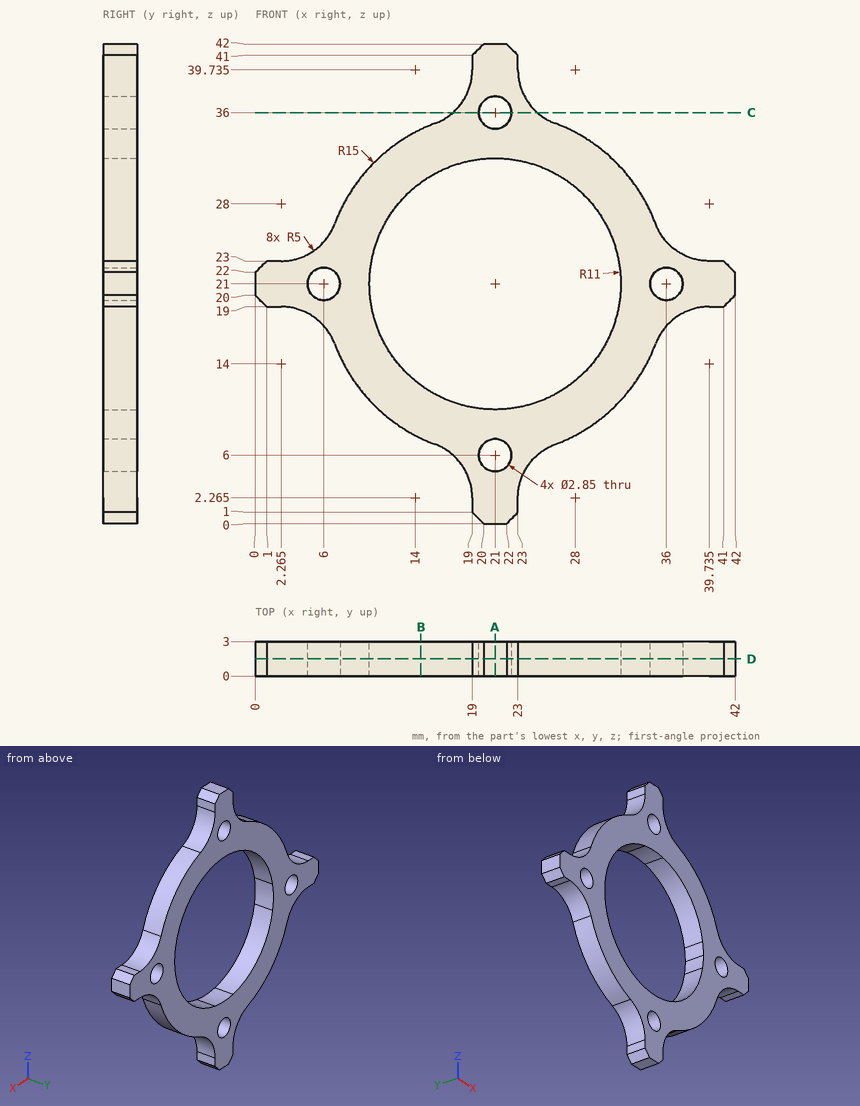
For this review, use the dimensioned drawing (mm, ordinates from the lowest corner) and the shaded views. Give positions to 0.01 mm unless a question says otherwise; leave off trailing zeros. Loops run counter-clockwise (first coordinate to the right, second up) from the corner with the lowest first, then second, coordinate; pieces in that order, holes last.
Item 1: Take a section at A-A, the plane x = 21. State the section outline as (y, z) points (3 decimals).
Item 2: For line 1 along X through (y, z) = (2.4, 21) (3 decimals); line 2 along X through (y, z) = (2.05, 22.5), list the stretches that pass through material, from the lowest coordinate up.
Item 3: Take a section at B-B, the plane x = 14.5. State the section outline as (y, z) points, and give its area (3 significant figures).
Item 4: Take a section at D-D, the plane y = 1.5. Give the number of separate pieces and of enclosed holes in the cut face, and give its area (3 significant figures).
Item 5: Insertion check: pin 1 (0.6 mm diameter, centred on y = 1.5, z = 40.5, fed in from +X); pin 2 (1.4 mm diameter, centred on x = 1.5, y = 2, fed in from +Z); pin 3 (1.4 mm diameter, centred on x = 1.5, y = 1.5, fed in from -Z). Each pin has a flat end and moves straight along its axis. Give the tip position at first contact, or say it passes through.
Item 6: Take a section at C-C, the plane z = 36. State the section outline as (x, y) points (3 decimals), and give its area (3 significant figures).
Calculated:
1. outline: (0, 0) - (3, 0) - (3, 4.575) - (0, 4.575) - close; (0, 7.425) - (3, 7.425) - (3, 10) - (0, 10) - close; (0, 32) - (3, 32) - (3, 34.575) - (0, 34.575) - close; (0, 37.425) - (3, 37.425) - (3, 42) - (0, 42) - close
2. line 1: x = 0 to 4.575, 7.425 to 10, 32 to 34.575, 37.425 to 42
2. line 2: x = 0.5 to 10.1, 31.9 to 41.5
3. outline: (0, 7.48) - (3, 7.48) - (3, 12.13) - (0, 12.13) - close; (0, 29.87) - (3, 29.87) - (3, 34.52) - (0, 34.52) - close
3. area: 27.9 mm2
4. separate pieces: 1
4. enclosed holes: 5
4. area: 415 mm2
5. pin 1: stops at x = 23
5. pin 2: stops at z = 23
5. pin 3: stops at z = 19
6. outline: (17.324, 0) - (19.575, 0) - (19.575, 3) - (17.324, 3) - close; (22.425, 0) - (24.676, 0) - (24.676, 3) - (22.425, 3) - close
6. area: 13.5 mm2
